Autodesk Inventor part; units mm, degrees
ref_plane "YZ Plane" through (0, 0, 0) normal (1, 0, 0) x (0, 1, 0)
ref_plane "XZ Plane" through (0, 0, 0) normal (0, 1, 0) x (-1, 0, 0)
ref_plane "XY Plane" through (0, 0, 0) normal (0, 0, 1) x (1, 0, 0)
sketch "Sketch1" plane through (0, 0, 0) normal (1, 0, 0) x (0, 1, 0)
  line L0 (0, 0) -> (8.6, 0)
  line L1 (8.6, 0) -> (8.6, -2.75)
  line L2 (8.6, -2.75) -> (15.6, -2.75)
  line L3 (15.6, -2.75) -> (66.85, 10.5)
  line L4 (66.85, 10.5) -> (66.85, 19.5)
  line L5 (66.85, 19.5) -> (51.85, 19.5)
  line L6 (51.85, 19.5) -> (51.85, 118.5)
  line L7 (51.85, 118.5) -> (66.85, 118.5)
  line L8 (66.85, 118.5) -> (66.85, 127.5)
  line L9 (42.85, 21) -> (8, 2)
  line L10 (8, 2) -> (0, 2)
  line L11 (0, 2) -> (0, 0)
  line L12 (0, 70) -> (0, 77)
  line L13 (0, 77) -> (-2.75, 77)
  line L14 (-2.75, 77) -> (-2.75, 70)
  line L15 (0, 70) -> (35.85, 70)
  line L16 (35.85, 70) -> (42.85, 59)
  line L17 (42.85, 94) -> (35.85, 83)
  line L18 (35.85, 83) -> (35.85, 70) construction
  line L19 (42.85, 127.5) -> (42.85, 94)
  line L20 (42.85, 59) -> (42.85, 21)
  line L21 (42.85, 127.5) -> (66.85, 127.5)
  line L22 (-1.375, 77) -> (-1.375, 90) construction
  arc A0 (1.866, 92.3443) -> (-5.375, 90) centre (-1.375, 90) ccw
  line L23 (-5.375, 90) -> (-5.375, 70)
  line L24 (1.866, 92.3443) -> (8.625, 83)
  circle A1 centre (-1.375, 90) radius 1.5
  line L25 (35.85, 83) -> (8.625, 83)
  line L26 (-2.75, 70) -> (-5.375, 70)
  dimension "d0" = 2.75
  dimension "d1" = 8.6
  dimension "d2" = 7
  dimension "d3" = 2
  dimension "d4" = 43.25
  dimension "d6" = 15
  dimension "d7" = 99
  dimension "d8" = 9
  dimension "d14" = 19.5
  dimension "d16" = 8
  dimension "d25" = 9
  dimension "d27" = 2.75
  dimension "d29" = 8.6
  dimension "d34" = 7
  dimension "d36" = 9
  dimension "d37" = 9
  dimension "d38" = 7
  dimension "d39" = 35
  dimension "d56" = 8
  dimension "d57" = 3
  dimension "d59" = 10
  dimension "d61" = 38
  dimension "d77" = 13
  dimension "d78" = 75
  dimension "d79" = 13
  dimension "d81" = 2.625
extrude "Extrusion1" add sketch "Sketch1" along normal blind 4.3
sketch "Sketch2" plane through (4.3, 0, 0) normal (1, 0, 0) x (0, 0, -1)
  line L0 (-120.5, 47.225) -> (-105.5, 47.225)
  line L1 (-105.5, 47.225) -> (-105.5, 44.475)
  line L2 (-105.5, 44.475) -> (-120.5, 44.475)
  line L3 (-120.5, 44.475) -> (-120.5, 47.225)
  line L4 (-90.5, 47.225) -> (-75.5, 47.225)
  line L5 (-75.5, 47.225) -> (-75.5, 44.475)
  line L6 (-75.5, 44.475) -> (-90.5, 44.475)
  line L7 (-90.5, 44.475) -> (-90.5, 47.225)
  line L8 (-60.5, 47.225) -> (-45.5, 47.225)
  line L9 (-45.5, 47.225) -> (-45.5, 44.475)
  line L10 (-45.5, 44.475) -> (-60.5, 44.475)
  line L11 (-60.5, 44.475) -> (-60.5, 47.225)
  line L12 (-30.5, 47.225) -> (-15.5, 47.225)
  line L13 (-15.5, 47.225) -> (-15.5, 44.475)
  line L14 (-15.5, 44.475) -> (-30.5, 44.475)
  line L15 (-30.5, 44.475) -> (-30.5, 47.225)
  line L16 (-127.5, 66.85) -> (-127.5, 42.85)
  line L17 (-19.5, 51.85) -> (-118.5, 51.85)
  line L18 (-127.5, 42.85) -> (-94, 42.85)
  line L19 (-105.5, 45.85) -> (-104.169, 45.85) construction
  line L20 (-104.169, 45.85) -> (-104.169, 42.85) construction
  line L21 (-127.5, 42.85) -> (-94, 42.85)
  point P0 (0, 0)
  dimension "d43" = 7
  dimension "d44" = 2.75
  dimension "d46" = 15
  dimension "d47" = 30
  dimension "d48" = 30
  dimension "d49" = 15
  dimension "d50" = 15
  dimension "d51" = 15
  dimension "d52" = 30
  dimension "d72" = 3
extrude "Extrusion2" cut sketch "Sketch2" against normal blind 10
fillet "Fillet1" radius 10 1 edges at (2.15, 42.85, 21)
sketch "Sketch4" plane through (4.3, 0, 0) normal (1, 0, 0) x (0, 0, -1)
  line L0 (-19.5, 51.85) -> (-118.5, 51.85)
  line L1 (-77.875, 51.85) -> (-75.125, 51.85)
  line L2 (-75.125, 51.85) -> (-75.125, 48.85)
  line L3 (-75.125, 48.85) -> (-77.875, 48.85)
  line L4 (-77.875, 48.85) -> (-77.875, 51.85)
  line L5 (-90.5, 47.225) -> (-75.5, 47.225)
  line L6 (-77, -2.75) -> (-77, 0)
  point P0 (0, 0)
  dimension "d73" = 3
  dimension "d74" = 1.625
  dimension "d82" = 0.875
  dimension "d83" = 2.75
extrude "Extrusion4" cut sketch "Sketch4" against normal blind 10
properties part number "TrayPanelG"
CAD build for the part. Positions are in the model's coordinates, mm. A direction names the side the tool comes from. Round coordinates to 2 decimals unless told otherwise and drop trailing zeros. Loops run counter-clockwise (first coordinate to the right, second up) from the corner with the lowest first, then second, coordinate; pieces in that order, holes last. Notation, with made-up numbers: M -12.5,64 L -4.5,64 A22 cw -4.5,102 Z; hole C 8.25,-32.75 d4. An arc over 180 degrees is marked long. Use a Markdown table: item, result. Add a question column.
(1) Cut at B-B (x = 2.45). State how many separate pieces and enclosed holes the cut face has, and give its area (3 significant figures).
(2) Which spindle directions (+Z, -Z, +X, -X, +Y, -Y) get a long thin tool onto all of the face, cutting with end or side? Do faces 4 (the face through (2, 50, 77.875)), 5 (the face through (2, 4, 2)), 6 (the face through (2, 44.475, 53)). Say none if no direction does.
(3) Flat gauge pins, fed straight in: pin 1 (1 mm diameter, centred on x = 2, y = 4.5, fed in from -Z); pin 2 (1.6 mm diameter, centred on x = 1.5, z = 1.5, fed in from -Y); pin 3 (2 mm diameter, centred on x = 2.5, z = 111, fed in from -Y). Where does each tip first touch, or does it go through?
(4) Cut at C-C (z = 100). Give the cut face in (x, y), and give its area (3 significant figures).
(5) Cut at D-D (y = 39). Give the cut face in (x, z).
(6) Drill centre lines: line 1 (Y direction, x = 0.8, z = 106) (3 decimals); line 2 (Y direction, x = 3.1, z = 90) (3 decimals); line 3 (Y direction, x = 3.9, z = 87.5) (3 decimals). Where is each one in solid material? Low to high.
(7) Pull direction Z, two halves, no side cores. Call faces 1 (the face through (2, 59, 19.5)), 2 (the face through (2.12, 40.866, 3.782)), 3 (the face through (2.12, -2.674, 93.783)): +Z half, -Z half, draft (parallel to the pull), parting line (faces both ways), or undercut.
(8) Cut at A-A (y = 30.5). Give the cut face in (x, z), and give its area (3 significant figures).
Geometry says:
| question | item | result |
|---|---|---|
| 1 | separate pieces | 1 |
| 1 | enclosed holes | 5 |
| 1 | area | 2,430 mm² |
| 2 | face 4 | +X, -X, +Y |
| 2 | face 5 | +X, -X, -Y |
| 2 | face 6 | +X, -X |
| 3 | pin 1 | stops at z = 0 |
| 3 | pin 2 | stops at y = 0 |
| 3 | pin 3 | stops at y = 42.85 |
| 4 | outline | M 0,42.85 L 4.3,42.85 L 4.3,51.85 L 0,51.85 Z |
| 4 | area | 38.7 mm² |
| 5 | outline | M 0,3.3 L 4.3,3.3 L 4.3,19.05 L 0,19.05 Z; M 0,65.05 L 4.3,65.05 L 4.3,87.95 L 0,87.95 Z |
| 6 | line 1 | y = 42.85 to 44.475, 47.225 to 51.85 |
| 6 | line 2 | y = -5.375 to -2.875, 0.125 to 3.562, 40.305 to 44.475, 47.225 to 51.85 |
| 6 | line 3 | y = -5.375 to 5.37, 38.714 to 44.475, 47.225 to 51.85 |
| 7 | face 1 | undercut |
| 7 | face 2 | -Z half |
| 7 | face 3 | +Z half |
| 8 | outline | M 0,1.1 L 4.3,1.1 L 4.3,14.27 L 0,14.27 Z; M 0,70 L 4.3,70 L 4.3,83 L 0,83 Z |
| 8 | area | 113 mm² |
